Model file for the job. Use its own axes, mm. Face numbers are marked on the shaded views. A direction names the side the tool comes from. Give positions to 0.01 mm unless a question says otherwise; leave off trailing zeros. Loops run counter-clockwise (first coordinate to the right, second up) from the corner with the lowest first, then second, coordinate; pieces in that order, holes last. Notation, with made-up numbers: (20, 22) - (58, 22) arc R24 cw to (58, 47) - close; hole circle Ø5 at (9.5, 30). An arc over 180 degrees is marked (long way). Answer as CSV lines item,"result". Start each with the question number.
Item 1: Pull direction Y, two halves, no side cores. Call the marked faces 4, 5 and 6: pulls with the +Y half, pulls with the -Y half, needs draft (parallel to the pull), parting line crosses it, or undercut.
Item 2: Tool access for the marked faces 1, 2 and 3: list every direction of +Z, -Z, +X, -X, +Y, -Y with a clear straight run to the whole face (end or side of a thin tool).
Item 3: Saw through at D-D on x = -8. Give the cut face in (y, z), plus the area to 3 significant figures.
Item 4: Pin check, flat tips, straight feed: pin 1 (1.8 mm diameter, centred on x = 4.5, z = -1, fed in from -Y); pin 2 (10 mm diameter, centred on x = -17, z = -4.5, fed in from +Y); pin 3 (3 mm diameter, centred on y = 6.5, z = -2.5, fed in from -X); pin 4 (6.5 mm diameter, centred on y = -51, z = -16.5, fed in from -X). Stop position of each tip, or through.
Item 5: Saw through at B-B on y = -16. Give the cut face in (x, z), plus the area to 3 significant figures.
Item 6: Saw through at C-C on y = -51. Give the cut face in (x, z), plus the area to 3 significant figures.
Item 7: Drill centre lines: L1, parallel to Z at x = 2.3, y = -16; L2, parallel to Z at x = -27.5, y = -52; L3, parallel to X at y = 13, z = 10.5. Where is each one in solid material? Low to high. Write a range as from..to.
Item 8: Saw through at A-A on z = 0. Give the cut face in (x, y).
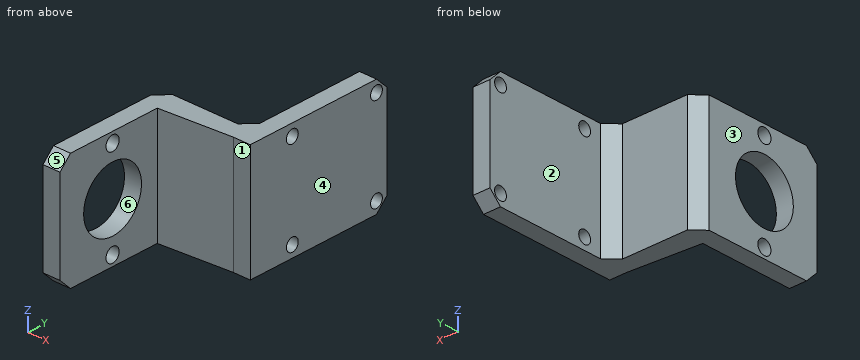
Autodesk Inventor part; units mm, degrees
ref_plane "YZ Plane" through (0, 0, 0) normal (1, 0, 0) x (0, 1, 0)
ref_plane "XZ Plane" through (0, 0, 0) normal (0, 1, 0) x (-1, 0, 0)
ref_plane "XY Plane" through (0, 0, 0) normal (0, 0, 1) x (1, 0, 0)
sketch "Skizze1" plane through (0, 0, 0) normal (1, 0, 0) x (0, 1, 0)
  line L0 (-20, -20) -> (20, -20)
  line L1 (20, -20) -> (20, 20)
  line L2 (20, 20) -> (-20, 20)
  line L3 (-20, 20) -> (-20, -20)
  line L4 (-20, -20) -> (20, 20) construction
  line L5 (20, -20) -> (-20, 20) construction
  line L6 (-16, -16) -> (16, -16) construction
  line L7 (16, -16) -> (16, 16) construction
  line L8 (16, 16) -> (-16, 16) construction
  line L9 (-16, 16) -> (-16, -16) construction
  line L10 (-16, -16) -> (16, 16) construction
  line L11 (16, -16) -> (-16, 16) construction
  circle A0 centre (16, 16) radius 2.25
  circle A1 centre (16, -16) radius 2.25
  circle A2 centre (-16, -16) radius 2.25
  circle A3 centre (-16, 16) radius 2.25
  line L12 (-20, 20) -> (-32, 20)
  line L13 (-32, 20) -> (-32, -20)
  line L14 (-32, -20) -> (-20, -20)
  line L15 (-20, -20) -> (-20, 20)
  point P0 (0, 0)
  dimension "d0" = 40
  dimension "d1" = 40
  dimension "d2" = 32
  dimension "d3" = 32
  dimension "d4" = 4.5
  dimension "d5" = 4.5
  dimension "d6" = 4.5
  dimension "d7" = 4.5
  dimension "d8" = 12
extrude "Extrusion1" add sketch "Skizze1" along normal blind 6
ref_plane "Arbeitsebene1" through (0, -32, 20) normal (0, 0, 1) x (1, 0, 0)
sketch "Skizze2" plane through (0, -32, 20) normal (0, 0, 1) x (1, 0, 0)
  line L0 (0, 52) -> (0, 0)
  line L1 (0, 0) -> (6, 0)
  line L2 (6, 52) -> (6, 0)
  line L3 (0, 52) -> (6, 52)
  line L4 (-31, 6) -> (-25, 6)
  line L5 (-25, 6) -> (-25, -39)
  line L6 (-25, -39) -> (-31, -39)
  line L7 (-31, -39) -> (-31, 6)
  line L8 (0, 0) -> (-25, -2)
  line L9 (-25, 6) -> (0, 6)
  point P0 (0, 32)
  point P1 (-28, -39)
  point P2 (-28, 6)
  dimension "d12" = 6
  dimension "d13" = 45
  dimension "d14" = 6
  dimension "d15" = 25
  dimension "d16" = 8
extrude "Extrusion2" add sketch "Skizze2" against normal up to surface (40 mm away) contours L0 L8 L5 L9 | L5 L6 L7 L4
chamfer "Fasen1" distance 4 angle 45 6 edges at (-31, -26, 0) (0, -26, 0) (-28, -71, -20) (-28, -71, 20) (3, 20, -20) (3, 20, 20)
sketch "Skizze3" plane through (-25, -34, 20) normal (1, 0, 0) x (0, 0, -1)
  line L0 (4, -37) -> (0, -33)
  line L1 (4, -37) -> (36, -37)
  line L2 (40, -33) -> (36, -37)
  line L3 (40, 0) -> (40, -33)
  line L4 (0, 0) -> (40, 0)
  line L5 (0, -33) -> (0, 0)
  circle A0 centre (20, -17) radius 20
  circle A1 centre (20, -17) radius 16.5
  point P0 (20, 34)
  dimension "d22" = 33
extrude "Extrusion3" cut sketch "Skizze3" along normal through all contours A1
sketch "Skizze4" plane through (-25, -67, 20) normal (1, 0, 0) x (0, 0, -1)
  line L0 (0, 33) -> (40, 33)
  line L1 (0, 0) -> (0, 33)
  line L2 (4, -4) -> (0, 0)
  line L3 (4, -4) -> (36, -4)
  line L4 (40, 0) -> (36, -4)
  line L5 (40, 33) -> (40, 0)
  circle A0 centre (20, 16) radius 16.5
  circle A1 centre (3.5, 16) radius 2.5
  circle A2 centre (36.5, 16) radius 2.5
  point P0 (20, 67)
  dimension "d25" = 5
  dimension "d26" = 5
extrude "Extrusion4" cut sketch "Skizze4" against normal blind 10 contours A0 A2 | A0 A2 | A1 A0 | A0 A1
sketch "Skizze5" plane through (-25, -67, 20) normal (1, 0, 0) x (0, 0, -1)
  line L0 (0, 35) -> (40, 35)
  line L1 (0, 33) -> (0, 35)
  line L2 (0, 33) -> (40, 33)
  circle A0 centre (20, 16) radius 11
  line L3 (40, 35) -> (40, 33)
  point P0 (20, 67)
  dimension "d29" = 22
extrude "Extrusion5" cut sketch "Skizze5" against normal blind 10 contours A0
properties part number "40_XYZstage_micrometer_motorized_nema8_samplemount_angle_distance_24mm"
Responses:
1,face 4,"needs draft"
1,face 5,"pulls with the -Y half"
1,face 6,"undercut"
2,face 1,"+Z, -Z, +X, -Y"
2,face 2,"+Z, -Z, -X, +Y"
2,face 3,"+Z, -Z, -X, +Y, -Y"
3,outline,"(-32.64, -20) - (-26, -20) - (-26, 20) - (-32.64, 20) - close"
3,area,"266 mm2"
4,pin 1,"y = -32"
4,pin 2,"y = -26"
4,pin 3,"x = 0"
4,pin 4,"x = -31"
5,outline,"(0, -20) - (6, -20) - (6, -18.25) - (0, -18.25) - close; (0, -13.75) - (6, -13.75) - (6, 13.75) - (0, 13.75) - close; (0, 18.25) - (6, 18.25) - (6, 20) - (0, 20) - close"
5,area,"186 mm2"
6,outline,"(-31, -20) - (-25, -20) - (-25, -19) - (-31, -19) - close; (-31, -14) - (-25, -14) - (-25, -11) - (-31, -11) - close; (-31, 11) - (-25, 11) - (-25, 14) - (-31, 14) - close; (-31, 19) - (-25, 19) - (-25, 20) - (-31, 20) - close"
6,area,"48.0 mm2"
7,L1,"-20..-18.25, -13.75..13.75, 18.25..20"
7,L2,"-20..-18.79, -14.21..-10.95, 10.95..14.21, 18.79..20"
7,L3,"0..6"
8,outline,"(-31, -71) - (-25, -71) - (-25, -62) - (-31, -62) - close; (-31, -40) - (-25, -40) - (-25, -34) - (0, -32) - (6, -32) - (6, 20) - (0, 20) - (0, -22) - (-4, -26) - (-27, -26) - (-31, -30) - close"
